Verification items for this drawing (mm, ordinates from the low corner). A direction names the side the tool comes from. Coordinates: 2 decimals unless noted, no trailing zeros. Order: outer loops, then holes, each group sorted by start corner. A loop starts at its lowest first (then second) coordinate and runs counter-clockwise, first axis right, second up. Notation, with made-up numbers: (-9.75, -37) -> (38.25, -37) arc R13 ccw to (38.25, -13) -> close; hole circle Ø4 at (75.25, -21.5). An arc over 180 degrees is marked (long way). Put each result on its own line as item: value. Start each with the question number.
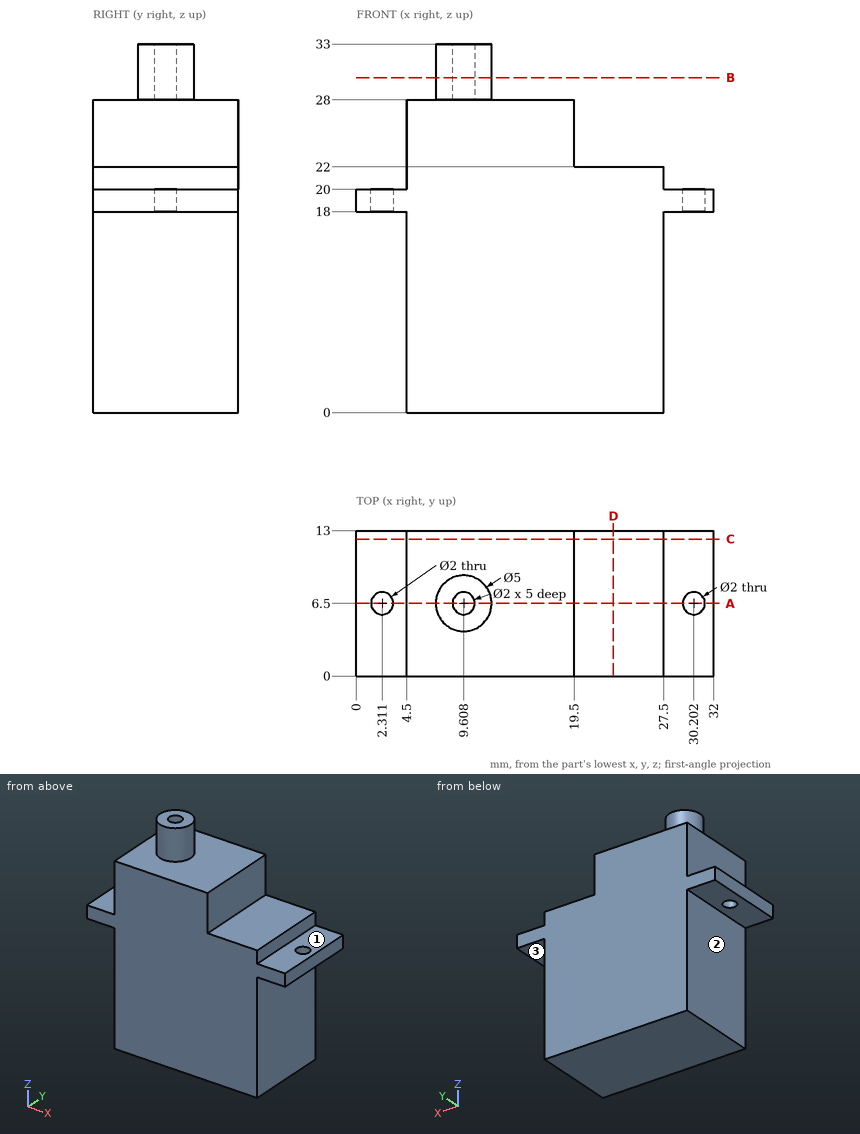
1) Sectioned sample at D-D (x = 23). Record the boundary of the cut face in (y, z), plus the area to 3 significant figures.
2) Sectioned sample at B-B (z = 30). Record the boundary of the cut face in (x, y), plus the area to 3 significant figures.
3) Scan lines: line 1 along Z through (x, y) = (21, 6.5); line 2 along Z through (x, y) = (6, 4); line 3 along X through (y, z) = (9.25, 24). Record each from-to range of solid material in increasing order. Write a range as [from, to].
4) Access from +Z, -Z, +X, -X, +Y, -Y to the whole of each face (thin tool, end or side, straight path). Record for the marked faces 1, 2 and 3.
5) Sectioned sample at A-A (y = 6.5). State how many separate pieces and enclosed holes the cut face has, plus the area to 3 significant figures.
6) Gauge pin test, flat ends, axial feed: pin 1 (1.3 mm diameter, centred on x = 30.5, y = 6.5, fed in from -Z); pin 2 (2 mm diameter, centred on x = 3, y = 7, fed in from -Z); pin 3 (5 mm diameter, centred on x = 29, y = 7.5, fed in from +Z); pin 4 (3 mm diameter, centred on y = 5, z = 25, fed in from +X). Record the tip position at first contact, or that the pin passes through.
7) Sectioned sample at C-C (y = 12.25). Record the boundary of the cut face in (x, z), plus the area to 3 significant figures.
Entries:
1. outline: (0, 0) -> (13, 0) -> (13, 22) -> (0, 22) -> close
1. area: 286 mm2
2. outline: circle Ø5 at (9.61, 6.5); hole circle Ø2 at (9.61, 6.5)
2. area: 16.5 mm2
3. line 1: z = [0, 22]
3. line 2: z = [0, 28]
3. line 3: x = [4.5, 19.5]
4. face 1: +Z, +X, +Y, -Y
4. face 2: -Z, -X, +Y, -Y
4. face 3: -Z, +X, +Y, -Y
5. separate pieces: 3
5. enclosed holes: 0
5. area: 621 mm2
6. pin 1: passes through
6. pin 2: stops at z = 18
6. pin 3: stops at z = 22
6. pin 4: stops at x = 19.5
7. outline: (0, 18) -> (4.5, 18) -> (4.5, 0) -> (27.5, 0) -> (27.5, 18) -> (32, 18) -> (32, 20) -> (27.5, 20) -> (27.5, 22) -> (19.5, 22) -> (19.5, 28) -> (4.5, 28) -> (4.5, 20) -> (0, 20) -> close
7. area: 614 mm2
